```python
from build123d import *

# Parameters (mm, degrees)
SKETCH1_W           = 267.603014698
SKETCH1_H           = 153.453144762
SKETCH1_R           = 2
SKETCH1_R_2         = 14.29
SKETCH1_R_3         = 2.499999953
SKETCH1_R_4         = 11
BOSS_EXTRUDE1_DEPTH = 4
SKETCH2_W           = 305.655174706
SKETCH2_H           = 186.291776367
CUT_EXTRUDE8_DEPTH  = 10


with BuildPart() as part:
    # Sketch1 → Boss-Extrude1 (new body)
    with BuildSketch(Plane.XY):
        with Locations((77.263379783, -10.843771022)):
            Rectangle(SKETCH1_W, SKETCH1_H)
        with Locations((-4.85811184, -43.49422294)):
            Circle(SKETCH1_R, mode=Mode.SUBTRACT)
        with Locations((101.811349412, -18.649052962)):
            Circle(SKETCH1_R_2, mode=Mode.SUBTRACT)
        with Locations((31.633252021, -61.264657987)):
            Circle(SKETCH1_R, mode=Mode.SUBTRACT)
        with Locations((10.251922178, 33.361755578)):
            Circle(SKETCH1_R, mode=Mode.SUBTRACT)
        with Locations((170.426367515, -60.775756941)):
            Circle(SKETCH1_R, mode=Mode.SUBTRACT)
        with Locations((161.513898191, 35.55251649)):
            Circle(SKETCH1_R, mode=Mode.SUBTRACT)
        with Locations((-4.85811184, 6.145317428)):
            Circle(SKETCH1_R, mode=Mode.SUBTRACT)
        with Locations((23.377209906, -42.310207828)):
            Circle(SKETCH1_R_3, mode=Mode.SUBTRACT)
        with Locations((23.377209906, -16.910207828)):
            Circle(SKETCH1_R_4, mode=Mode.SUBTRACT)
        with Locations((1.38016465, -29.610207828)):
            Circle(SKETCH1_R_3, mode=Mode.SUBTRACT)
        with Locations((1.38016465, -4.210207828)):
            Circle(SKETCH1_R_3, mode=Mode.SUBTRACT)
        with Locations((23.377209906, 8.489792172)):
            Circle(SKETCH1_R_3, mode=Mode.SUBTRACT)
        with Locations((45.374255162, -4.210207828)):
            Circle(SKETCH1_R_3, mode=Mode.SUBTRACT)
        with Locations((45.374255162, -29.610207828)):
            Circle(SKETCH1_R_3, mode=Mode.SUBTRACT)
    extrude(amount=BOSS_EXTRUDE1_DEPTH)

    # Sketch2 → Cut-Extrude8 (cut)
    # profile 1 of 11: a face of its own
    with BuildSketch(Plane.XY.offset(4)):
        with Locations((67.603615112, -0.467239306)):
            Rectangle(SKETCH2_W, SKETCH2_H)
        with BuildLine():
            Line((15.316933469, 37.435532771), (156.333033267, 39.477900374))
            ThreePointArc((156.333033267, 39.477900374), (159.128219206, 41.598881992), (162.618590728, 41.957955929))
            ThreePointArc((162.618590728, 41.957955929), (163.868628825, 41.61100175), (165.024869365, 41.022715885))
            ThreePointArc((165.024869365, 41.022715885), (167.217901725, 38.66930068), (168.013898191, 35.55251649))
            ThreePointArc((168.013898191, 35.55251649), (167.480787607, 32.974488039), (165.968904131, 30.819343974))
            Line((165.968904131, 30.819343974), (173.937338688, -55.305557546))
            ThreePointArc((173.937338688, -55.305557546), (176.130371049, -57.658972751), (176.926367515, -60.775756941))
            ThreePointArc((176.926367515, -60.775756941), (172.552302777, -66.918264512), (165.317013897, -64.79377954))
            Line((165.317013897, -64.79377954), (36.770785596, -65.246585756))
            ThreePointArc((36.770785596, -65.246585756), (28.080665231, -66.707922367), (25.920047751, -58.164771381))
            Line((25.920047751, -58.164771381), (21.755974451, -48.604776567))
            ThreePointArc((21.755974451, -48.604776567), (19.929745718, -47.82065161), (18.425821295, -46.521353851))
            Line((18.425821295, -46.521353851), (0.428452826, -47.276052396))
            ThreePointArc((0.428452826, -47.276052396), (-9.356992337, -48.185712497), (-8.85811184, -38.370747557))
            Line((-8.85811184, -38.370747557), (-8.85811184, 1.021842045))
            ThreePointArc((-8.85811184, 1.021842045), (-11.150528938, 7.774883952), (-5.868402241, 12.566323058))
            Line((-5.868402241, 12.566323058), (4.267840814, 30.823888318))
            ThreePointArc((4.267840814, 30.823888318), (3.803217243, 34.176743104), (5.087377177, 37.308586577))
            ThreePointArc((5.087377177, 37.308586577), (6.293465571, 38.517395333), (7.772745355, 39.370389556))
            ThreePointArc((7.772745355, 39.370389556), (11.866714012, 39.657980425), (15.316933469, 37.435532771))
        make_face(mode=Mode.SUBTRACT)
    # profile 2 of 11: a face of its own
    with BuildSketch(Plane.XY.offset(4)):
        with BuildLine():
            Line((87.009313409, 30.473030477), (25.016174455, 29.575170029))
            Line((25.016174455, 29.575170029), (84.534856694, -4.234726778))
            ThreePointArc((84.534856694, -4.234726778), (88.475465617, -0.527126923), (93.187242807, 2.132544312))
            Line((93.187242807, 2.132544312), (87.009313409, 30.473030477))
        make_face()
    # profile 3 of 11: a face of its own
    with BuildSketch(Plane.XY.offset(4)):
        with BuildLine():
            Line((115.516142216, -0.804483643), (150.988719582, 31.399658477))
            Line((150.988719582, 31.399658477), (95.171415855, 30.591244026))
            Line((95.171415855, 30.591244026), (101.003681787, 3.83644621))
            ThreePointArc((101.003681787, 3.83644621), (108.66470749, 2.781800569), (115.516142216, -0.804483643))
        make_face()
    # profile 4 of 11: a face of its own
    with BuildSketch(Plane.XY.offset(4)):
        with BuildLine():
            Line((158.26921014, 27.20426024), (120.893532253, -6.72763115))
            ThreePointArc((120.893532253, -6.72763115), (122.397082717, -9.567335928), (123.480802665, -12.592255482))
            Line((123.480802665, -12.592255482), (161.619207477, -9.003377368))
            Line((161.619207477, -9.003377368), (158.26921014, 27.20426024))
        make_face()
    # profile 5 of 11: a face of its own
    with BuildSketch(Plane.XY.offset(4)):
        with BuildLine():
            Line((122.77328809, -26.825062188), (165.706925432, -53.184490212))
            Line((165.706925432, -53.184490212), (162.356235259, -16.969364249))
            Line((162.356235259, -16.969364249), (124.230302911, -20.557068686))
            ThreePointArc((124.230302911, -20.557068686), (123.727037564, -23.743423664), (122.77328809, -26.825062188))
        make_face()
    # profile 6 of 11: a face of its own
    with BuildSketch(Plane.XY.offset(4)):
        with BuildLine():
            Line((94.560961812, -57.042969272), (156.346956485, -56.825327083))
            Line((156.346956485, -56.825327083), (118.587568032, -33.642667897))
            ThreePointArc((118.587568032, -33.642667897), (109.853001514, -39.662901526), (99.330831485, -41.011902307))
            Line((99.330831485, -41.011902307), (94.560961812, -57.042969272))
        make_face()
    # profile 7 of 11: a face of its own
    with BuildSketch(Plane.XY.offset(4)):
        with BuildLine():
            Line((84.962067713, -33.560515205), (46.010236401, -57.213990006))
            Line((46.010236401, -57.213990006), (86.20559517, -57.072401189))
            Line((86.20559517, -57.072401189), (91.663047334, -38.730436503))
            ThreePointArc((91.663047334, -38.730436503), (88.067281455, -36.463389772), (84.962067713, -33.560515205))
        make_face()
    # profile 8 of 11: a face of its own
    with BuildSketch(Plane.XY.offset(4)):
        with BuildLine():
            ThreePointArc((80.809710516, -26.722538187), (80.077925828, -24.47213628), (79.586542538, -22.157323106))
            Line((79.586542538, -22.157323106), (53.013387432, -21.568209721))
            ThreePointArc((53.013387432, -21.568209721), (46.235949771, -36.339001197), (32.750489376, -45.408306571))
            Line((32.750489376, -45.408306571), (34.506149029, -54.840346462))
            Line((34.506149029, -54.840346462), (80.809710516, -26.722538187))
        make_face()
    # profile 9 of 11: a face of its own
    with BuildSketch(Plane.XY.offset(4)):
        with BuildLine():
            ThreePointArc((79.763854917, -14.159288328), (80.122803307, -12.660984172), (80.583447278, -11.190757516))
            Line((80.583447278, -11.190757516), (16.516137359, 25.203010887))
            Line((16.516137359, 25.203010887), (19.736612333, 12.868073675))
            ThreePointArc((19.736612333, 12.868073675), (41.978293765, 6.62698995), (53.190699811, -13.570174942))
            Line((53.190699811, -13.570174942), (79.763854917, -14.159288328))
        make_face()
    # profile 10 of 11: a face of its own
    with BuildSketch(Plane.XY.offset(4)):
        with BuildLine():
            Line((11.996082824, 10.847132577), (8.903504201, 22.692206192))
            Line((8.903504201, 22.692206192), (1.125969524, 8.683184687))
            ThreePointArc((1.125969524, 8.683184687), (1.511602787, 7.440205673), (1.64188816, 6.145317428))
            ThreePointArc((1.64188816, 6.145317428), (1.374954172, 4.30171007), (0.59607644, 2.609524701))
            ThreePointArc((0.59607644, 2.609524701), (5.806508232, 7.405845361), (11.996082824, 10.847132577))
        make_face()
    # profile 11 of 11: a face of its own
    with BuildSketch(Plane.XY.offset(4)):
        with BuildLine():
            Line((-0.85811184, -34.592096299), (-0.85811184, -38.370747557))
            ThreePointArc((-0.85811184, -38.370747557), (-0.359231342, -38.802733382), (0.093276771, -39.283076917))
            Line((0.093276771, -39.283076917), (3.243928256, -39.150958041))
            ThreePointArc((3.243928256, -39.150958041), (1.076110226, -36.976621387), (-0.85811184, -34.592096299))
        make_face()
    extrude(amount=-CUT_EXTRUDE8_DEPTH, mode=Mode.SUBTRACT)


solid = part.part
```
The model under review builds one solid part; all positions refer to its coordinate system, in mm. Give positions to 0.01 mm unless a question says otherwise; leave off trailing zeros. Write each loop counter-clockwise with the first axis right and the second up, starting at its lowest first coordinate (ties: lowest second). Pieces come first, ordered by that corner, then holes. Notation, with made-up numbers: M -12.5,4.5 L -7.5,4.5 A21 cw -7.5,42.5 Z; hole C -21,-37 d8. An arc over 180 degrees is marked long. Write item = value, one per line. Start each with the question number.
Q1. We need section A-A (y = 16.5). State the section outline as (x, z) points, plus the area to 3 significant figures.
Q2. We need section B-B (z = 1.05). Give the number of separate pieces and of enclosed holes in the cut face, plus the area to 3 significant figures.
Q3. For line 1 (X direction, y = -61, z = 1.65); line 2 (X direction, y = -35, z = 3.1); line 3 (Y direction, x = 154, z = 3), list the stretches that pass through material, from the lowest coordinate up.
Q4. Clearance check with flat-ended pins moving along their axes: pin 1 (1.1 mm diameter, centred on y = -36.5, z = 1.5, fed in from +X); pin 2 (2 mm diameter, centred on x = 12, z = 1.5, fed in from -Y); pin 3 (2 mm diameter, centred on x = 87.5, z = 1, fed in from +Y); pin 4 (23 mm diameter, centred on x = 101.81, y = -18.65, fed in from -Z). State where each tip first meets the part, or that it passes through.
Q5. Mouldability with a two-part tool opening along X and no side actions: class faces 1 (the face through (-8.858, -19, 2)), 2 (the face through (81, -12, 4)), 3 (the face through (143.56, -18.74, 2.03)) as released by +X, released by -X, zero draft, split by the parting line, or undercut.
Result set:
q1.outline = M -3.68,0 L 5.47,0 L 5.47,4 L -3.68,4 Z; M 10.52,0 L 18.79,0 L 18.79,4 L 10.52,4 Z; M 31.84,0 L 48.03,0 L 48.03,4 L 31.84,4 Z; M 90.06,0 L 98.24,0 L 98.24,4 L 90.06,4 Z; M 134.58,0 L 146.48,0 L 146.48,4 L 134.58,4 Z; M 159.26,0 L 167.29,0 L 167.29,4 L 159.26,4 Z
q1.area = 247 mm2
q2.separate_pieces = 1
q2.enclosed_holes = 24
q2.area = 10,100 mm2
q3.line_1 = 25.14 to 29.65, 33.62 to 168.44, 172.41 to 176.92
q3.line_2 = -8.86 to -0.86, -0.56 to 47.31, 67.18 to 82.59, 86.36 to 117.27, 120.8 to 136.09, 164.02 to 172.06
q3.line_3 = -64.83 to -56.83, -55.38 to -46, -17.76 to -9.72, 23.33 to 39.44
q4.pin_1 = 172.25
q4.pin_2 = -46.83
q4.pin_3 = 38.5
q4.pin_4 = through
q5.face_1 = released by -X
q5.face_2 = zero draft
q5.face_3 = undercut
